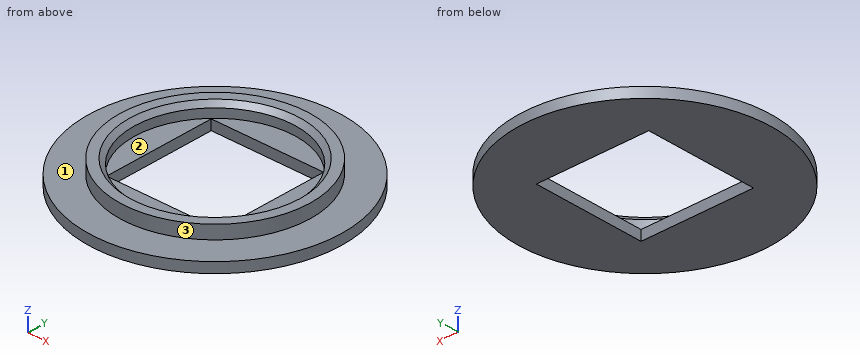
from build123d import *

# Parameters (mm, degrees)
SKETCH_1_R          = 8
EXTRUDE_1_DEPTH     = 0.65
EXTRUDE_START       = 0.65
SKETCH_2_R          = 6.02
SKETCH_2_R_2        = 5.1
EXTRUDE_2_DEPTH     = 0.85
CUT_EXTRUDE_START   = 0.65
SKETCH_3_R          = 5.1
CUT_EXTRUDE_1_DEPTH = 0.01
CUT_EXTRUDE_2_DEPTH = 0.64
CHAMFER_1_SIZE      = 0.3


with BuildPart() as part:
    # 草图1 → 凸台-拉伸1 (new body)
    with BuildSketch(Plane.XY):
        Circle(SKETCH_1_R)
    extrude(amount=EXTRUDE_1_DEPTH)

    # 草图2 → 凸台-拉伸2 (add)
    with BuildSketch(Plane.XY.offset(EXTRUDE_START)):
        Circle(SKETCH_2_R)
        Circle(SKETCH_2_R_2, mode=Mode.SUBTRACT)
    extrude(amount=EXTRUDE_2_DEPTH)

    # 草图3 → 切除-拉伸1 (cut)
    with BuildSketch(Plane.XY.offset(CUT_EXTRUDE_START)):
        Circle(SKETCH_3_R)
    extrude(amount=-CUT_EXTRUDE_1_DEPTH, mode=Mode.SUBTRACT)

    # 草图4 → 切除-拉伸2 (cut)
    with BuildSketch(Plane.XY):
        Polygon((-3.57, 3.57), (3.57, 3.57), (3.57, -3.57), (-3.57, -3.57), (-3.57, 0), align=None)
    extrude(amount=CUT_EXTRUDE_2_DEPTH, mode=Mode.SUBTRACT)

    # 倒角1
    chamfer_1_edges = [part.edges().sort_by_distance(p)[0] for p in [
        (-5.1, 0, 1.5),
    ]]
    chamfer(chamfer_1_edges, length=CHAMFER_1_SIZE)


solid = part.part
Can you work these out from the model? Positions are in its coordinate system, mm. Face numbers are marked on the shaded views. Coordinates: 2 decimals unless noted, no trailing zeros. Write each loop counter-clockwise with the first axis right and the second up, starting at its lowest first coordinate (ties: lowest second). Pieces come first, ordered by that corner, then holes. Notation, with made-up numbers: (36, 70) -> (80, 70) arc R24 ccw to (80, 92) -> close; hole circle Ø6 at (59.5, -5). An arc over 180 degrees is marked (long way). Write each question's results on one line, items separated by ' | '. Start each with the question number.
Q1. Imagine slicing it at C-C (z = 0.4). Write out the boundary of the cut face in (x, y), then the cut area to 3 significant figures.
Q2. I'm going to push a flat-ended pin straight in: pin 1 (8 mm diameter, centred on x = 0, y = -0.5, fed in from +Z). Where does the tip first touch, or does it pass through?
Q3. Imagine slicing it at A-A (x = 0). Write out the boundary of the cut face in (y, z).
Q4. Imagine slicing it at D-D (x = -6.5). Write out the boundary of the cut face in (y, z), then the cut area to 3 significant figures.
Q5. If I drill on probe 1 along Y at (x, z) = (0, 0.8); probe 2 along X at (y, z) = (0.25, 0.35); probe 3 along Z at (x, y) = (1, -6.75), over which ranges is the centre line in solid material (lowest first)?
Q6. We'd pull the mould along X, two halves only. Please class the marked faces 1, 2 and 3: +X half, -X half, draft (parallel to the pull), parting line (faces both ways), or undercut.
Taken from the geometry:
1) outline: circle Ø16 at (0, 0); hole (-3.57, -3.57) -> (3.57, -3.57) -> (3.57, 3.57) -> (-3.57, 3.57) -> close | area: 150 mm^2
2) pin 1: stops at z = 0.64
3) outline: (-8, 0) -> (-3.57, 0) -> (-3.57, 0.64) -> (-5.1, 0.64) -> (-5.1, 1.2) -> (-5.4, 1.5) -> (-6.02, 1.5) -> (-6.02, 0.65) -> (-8, 0.65) -> close; (3.57, 0) -> (8, 0) -> (8, 0.65) -> (6.02, 0.65) -> (6.02, 1.5) -> (5.4, 1.5) -> (5.1, 1.2) -> (5.1, 0.64) -> (3.57, 0.64) -> close
4) outline: (-4.66, 0) -> (4.66, 0) -> (4.66, 0.65) -> (-4.66, 0.65) -> close | area: 6.06 mm^2
5) probe 1: y = -6.02 to -5.1, 5.1 to 6.02 | probe 2: x = -8 to -3.57, 3.57 to 8 | probe 3: z = 0 to 0.65
6) face 1: draft | face 2: undercut | face 3: parting line
